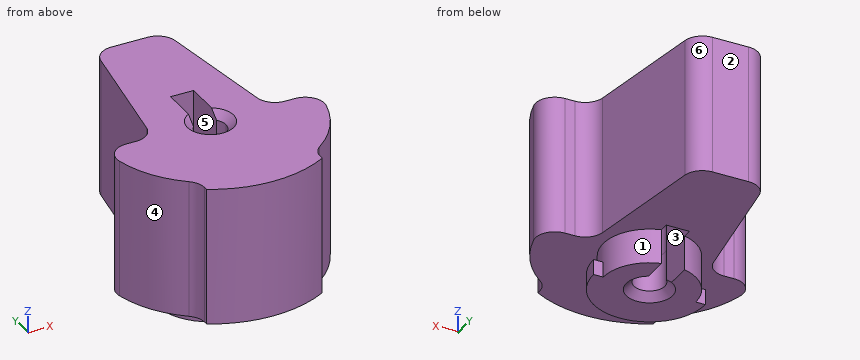
```python
from build123d import *

# Parameters (mm, degrees)
BOSS_EXTRUDE2_DEPTH  = 9.144
CUT_EXTRUDE1_DEPTH   = 0.508
SKETCH4_W            = 1.524
SKETCH4_H            = 3.556
CUT_EXTRUDE2_DEPTH   = 10.144
BOSS_EXTRUDE8_DEPTH  = 9.144
BOSS_EXTRUDE10_DEPTH = 9.144
FILLET2_R            = 1.27
CUT_EXTRUDE4_DEPTH   = 9.144
FILLET4_R            = 1.27
BOSS_EXTRUDE11_DEPTH = 1.27
BOSS_EXTRUDE12_DEPTH = 1.016
BOSS_EXTRUDE13_START = -0.508
BOSS_EXTRUDE13_DEPTH = 0.508
BOSS_EXTRUDE14_DEPTH = 1.27
BOSS_EXTRUDE15_DEPTH = 1.016


with BuildPart() as part:
    # Sketch2 → Boss-Extrude2 (new body)
    with BuildSketch(Plane.XY):
        with BuildLine():
            ThreePointArc((-3.81, 0), (0, -3.81), (3.81, 0))
            Line((3.81, 0), (3.81, 8.636))
            ThreePointArc((3.81, 8.636), (3.363630735, 9.713630735), (2.286, 10.16))
            Line((2.286, 10.16), (-2.286, 10.16))
            ThreePointArc((-2.286, 10.16), (-3.363630735, 9.713630735), (-3.81, 8.636))
            Line((-3.81, 8.636), (-3.81, 0))
        make_face()
        with BuildLine():
            Line((-0.762, 0), (1.016, 0))
            ThreePointArc((1.016, 0), (-0.359210245, -0.950380976), (-0.762, 0.672020833))
            Line((-0.762, 0.672020833), (-0.762, 0))
        make_face(mode=Mode.SUBTRACT)
    extrude(amount=BOSS_EXTRUDE2_DEPTH)

    # Sketch3 → Cut-Extrude1 (cut)
    with BuildSketch(Plane.XY.offset(9.144)):
        with BuildLine():
            Line((-0.762, 0), (1.016, 0))
            ThreePointArc((1.016, 0), (0.950380976, 0.359210245), (0.762, 0.672020833))
            Line((0.762, 0.672020833), (0.762, 3.556))
            Line((0.762, 3.556), (-0.762, 3.556))
            Line((-0.762, 3.556), (-0.762, 0))
        make_face()
    extrude(amount=-CUT_EXTRUDE1_DEPTH, mode=Mode.SUBTRACT)

    # Sketch4 → Cut-Extrude2 (cut, through all)
    with BuildSketch(Plane(origin=(0, 0, 0), x_dir=(-1, 0, 0), z_dir=(0, 0, -1))):
        with Locations((0, 1.778)):
            Rectangle(SKETCH4_W, SKETCH4_H)
    extrude(amount=-CUT_EXTRUDE2_DEPTH, mode=Mode.SUBTRACT)

    # Sketch7 → Cut-Revolve1 (revolve, cut)
    with BuildSketch(Plane(origin=(0, 0, 0), x_dir=(1, 0, 0), z_dir=(0, 1, 0))):
        Polygon((0, 0), (0, -9.144), (1.524, -9.144), (1.016, -8.636), (1.016, -0.508), (1.524, 0), align=None)
    revolve(axis=Axis((0, 0, 0), (0, 0, 1)), mode=Mode.SUBTRACT)

    # Sketch10 → Boss-Extrude8 (add)
    with BuildSketch(Plane.XY.offset(9.144)):
        with BuildLine():
            Line((-3.81, 0), (-6.985, 0))
            ThreePointArc((-6.985, 0), (0, -6.985), (6.985, 0))
            Line((6.985, 0), (3.81, 0))
            ThreePointArc((3.81, 0), (0, -3.81), (-3.81, 0))
        make_face()
    extrude(amount=-BOSS_EXTRUDE8_DEPTH)

    # Sketch14 → Boss-Extrude10 (add)
    with BuildSketch(Plane.XY.offset(9.144)):
        with BuildLine():
            ThreePointArc((3.81, -5.85441073), (0, -6.985), (-3.81, -5.85441073))
            Line((-3.81, -5.85441073), (-3.81, -6.745362036))
            ThreePointArc((-3.81, -6.745362036), (0, -7.747), (3.81, -6.745362036))
            Line((3.81, -6.745362036), (3.81, -5.85441073))
        make_face()
    extrude(amount=-BOSS_EXTRUDE10_DEPTH)

    # Fillet2
    fillet2_edges = [part.edges().sort_by_distance(p)[0] for p in [
        (6.985, 0, 4.572),
        (-6.985, 0, 4.572),
    ]]
    fillet(fillet2_edges, radius=FILLET2_R)

    # Sketch16 → Cut-Extrude4 (cut)
    with BuildSketch(Plane.XY.offset(9.144)):
        with BuildLine():
            Line((-3.81, 0), (-2.286, 10.16))
            ThreePointArc((-2.286, 10.16), (-3.363630735, 9.713630735), (-3.81, 8.636))
            Line((-3.81, 8.636), (-3.81, 0))
        make_face()
        with BuildLine():
            Line((2.286, 10.16), (3.81, 0))
            Line((3.81, 0), (3.81, 8.636))
            ThreePointArc((3.81, 8.636), (3.363630735, 9.713630735), (2.286, 10.16))
        make_face()
    extrude(amount=-CUT_EXTRUDE4_DEPTH, mode=Mode.SUBTRACT)

    # Fillet4
    fillet4_edges = [part.edges().sort_by_distance(p)[0] for p in [
        (-3.81, -5.85441073, 4.572),
        (3.81, -5.85441073, 4.572),
        (-3.81, 0, 4.572),
        (-2.286, 10.16, 4.572),
        (2.286, 10.16, 4.572),
        (3.81, 0, 4.572),
    ]]
    fillet(fillet4_edges, radius=FILLET4_R)

    # Sketch17 → Boss-Extrude11 (add)
    with BuildSketch(Plane(origin=(0, 0, 0), x_dir=(-1, 0, 0), z_dir=(0, 0, -1))):
        with BuildLine():
            Line((0.762, 2.95121331), (0.762, 1.319822715))
            ThreePointArc((0.762, 1.319822715), (0, -1.524), (-0.762, 1.319822715))
            Line((-0.762, 1.319822715), (-0.762, 2.95121331))
            ThreePointArc((-0.762, 2.95121331), (-1.866511184, -2.409655577), (3.048, 0))
            ThreePointArc((3.048, 0), (2.409655577, 1.866511184), (0.762, 2.95121331))
        make_face()
    extrude(amount=BOSS_EXTRUDE11_DEPTH)

    # Sketch18 → Boss-Extrude12 (add)
    with BuildSketch(Plane(origin=(0, 0, -1.27), x_dir=(-1, 0, 0), z_dir=(0, 0, -1))):
        with BuildLine():
            Line((-1.524, 0), (-3.048, 0))
            ThreePointArc((-3.048, 0), (0, -3.048), (3.048, 0))
            Line((3.048, 0), (1.524, 0))
            ThreePointArc((1.524, 0), (0, -1.524), (-1.524, 0))
        make_face()
        with BuildLine():
            Line((-3.048, 0), (-3.683, 0))
            ThreePointArc((-3.683, 0), (0, -3.683), (3.683, 0))
            Line((3.683, 0), (3.048, 0))
            ThreePointArc((3.048, 0), (0, -3.048), (-3.048, 0))
        make_face()
    extrude(amount=BOSS_EXTRUDE12_DEPTH)

    # Sketch20 → Boss-Extrude13 (add)
    with BuildSketch(Plane(origin=(0, 0, 0), x_dir=(-1, 0, 0), z_dir=(0, 0, -1)).offset(BOSS_EXTRUDE13_START)):
        with BuildLine():
            Line((0.762, 1.319822715), (0.762, 0.672020833))
            ThreePointArc((0.762, 0.672020833), (0, -1.016), (-0.762, 0.672020833))
            Line((-0.762, 0.672020833), (-0.762, 1.319822715))
            ThreePointArc((-0.762, 1.319822715), (0, -1.524), (0.762, 1.319822715))
        make_face()
    extrude(amount=BOSS_EXTRUDE13_DEPTH)

    # Sketch21 → Boss-Extrude14 (add)
    with BuildSketch(Plane(origin=(0, 0, 0), x_dir=(-1, 0, 0), z_dir=(0, 0, -1))):
        with BuildLine():
            Line((0.762, 1.319822715), (0.762, 0.672020833))
            ThreePointArc((0.762, 0.672020833), (0, -1.016), (-0.762, 0.672020833))
            Line((-0.762, 0.672020833), (-0.762, 1.319822715))
            ThreePointArc((-0.762, 1.319822715), (0, -1.524), (0.762, 1.319822715))
        make_face()
    extrude(amount=BOSS_EXTRUDE14_DEPTH)

    # Sketch22 → Boss-Extrude15 (add)
    with BuildSketch(Plane(origin=(0, 0, -1.27), x_dir=(-1, 0, 0), z_dir=(0, 0, -1))):
        with BuildLine():
            Line((0.762, 2.95121331), (0.762, 0.672020833))
            ThreePointArc((0.762, 0.672020833), (0, -1.016), (-0.762, 0.672020833))
            Line((-0.762, 0.672020833), (-0.762, 2.95121331))
            ThreePointArc((-0.762, 2.95121331), (-2.409655577, 1.866511184), (-3.048, 0))
            Line((-3.048, 0), (-1.524, 0))
            ThreePointArc((-1.524, 0), (0, -1.524), (1.524, 0))
            Line((1.524, 0), (3.048, 0))
            ThreePointArc((3.048, 0), (2.409655577, 1.866511184), (0.762, 2.95121331))
        make_face()
    extrude(amount=BOSS_EXTRUDE15_DEPTH)

    # Sketch23 → Cut-Revolve2 (revolve, cut)
    with BuildSketch(Plane(origin=(0, 0, 0), x_dir=(1, 0, 0), z_dir=(0, 1, 0))):
        Polygon((0, 2.286), (0, 0), (0.762, 0), (0.762, 1.524), (1.524, 2.286), align=None)
    revolve(axis=Axis((0, 0, -2.286), (0, 0, 1)), mode=Mode.SUBTRACT)


solid = part.part
```
For this review, take the finished solid that the model builds, in its own axes (mm). Face numbers are marked on the shaded views. A direction names the side the tool comes from. Coordinates: 2 decimals unless noted, no trailing zeros. Loops run counter-clockwise (first coordinate to the right, second up) from the corner with the lowest first, then second, coordinate; pieces in that order, holes last. Notation, with made-up numbers: (61, 30) - (81, 30) arc R18 ccw to (81, 65) - close; hole circle Ø1 at (77.5, 74). An arc over 180 degrees is marked (long way). Use one line per item in the form item = value. Start each with the question number.
1) For the marked faces 1 and 2, list the 3-axis set-ups (+Z, -Z, +X, -X, +Y, -Y) from which the entire face can be reached by the end or side of a thin tool; tool diameter is ignored.
2) Take a section at C-C (z = 4.75). State the section outline as (x, y) points (3 decimals).
3) For pin 1 (0.5 mm diameter, centred on x = -5, z = 6, fed in from +Y); pin 2 (1 mm diameter, centred on x = -3, z = 1.5, fed in from -Y); pin 3 (0.7 mm diameter, centred on x = 3, z = -2, fed in from +Y), all flat-tipped, find the tip position at first contact; note any pin that passes through.
4) To check wall thickness, follow probe 1 along X at (y, z) = (0, -0.8); probe 2 along Y at (x, z) = (0, -0.35); probe 3 along Z at (x, y) = (1, -3.75). State the ranges of each line that lie inside material, in increasing order. Write a range as from..to.
5) Draft analysis for pull direction X (two halves, no side actions). For the marked faces 3, 4, 5 and 6, state which applies: released by +X, released by -X, zero draft, split by the parting line, or undercut.
6) Take a section at B-B (y = 3.25). State the section outline as (x, z) points.
7) Take a section at D-D (z = -1.5). State the section outline as (x, y) points, plus the area to 3 significant figures.
8) Take a section at A-A (x = 0). State the section outline as (y, z) points, plus the area to 3 significant figures.
From the geometry:
q1.face_1 = none
q1.face_2 = +Z, -Z, +X, -X, +Y
q2.outline = (-6.81, -1.552) arc R6.985 ccw to (-4.298, -5.506) arc R1.27 cw to (-3.81, -6.507) - (-3.81, -6.745) arc R7.747 ccw to (3.81, -6.745) - (3.81, -6.507) arc R1.27 cw to (4.298, -5.506) arc R6.985 ccw to (6.81, -1.552) arc R1.27 ccw to (5.572, 0) - (4.904, 0) arc R1.27 cw to (3.648, 1.082) - (2.448, 9.078) arc R1.27 ccw to (1.192, 10.16) - (-1.192, 10.16) arc R1.27 ccw to (-2.448, 9.078) - (-3.648, 1.082) arc R1.27 cw to (-4.904, 0) - (-5.572, 0) arc R1.27 ccw to start; hole (-0.762, 0.672) arc R1.016 ccw (long way) to (0.762, 0.672) - (0.762, 3.556) - (-0.762, 3.556) - close
q3.pin_1 = 0.01
q3.pin_2 = -7.33
q3.pin_3 = 1.51
q4.probe_1 = -3.05..-1.02, 1.02..3.05
q4.probe_2 = -3.05..-1.02
q4.probe_3 = 0..9.14
q5.face_3 = undercut
q5.face_4 = released by -X
q5.face_5 = undercut
q5.face_6 = released by +X
q6.outline = (-3.32, 0) - (-0.76, 0) - (-0.76, 9.14) - (-3.32, 9.14) - close; (0.76, 0) - (3.32, 0) - (3.32, 9.14) - (0.76, 9.14) - close
q7.outline = (-3.68, 0) arc R3.68 ccw to (3.68, 0) - (3.05, 0) arc R3.05 ccw to (0.76, 2.95) - (0.76, 0.67) arc R1.02 cw (long way) to (-0.76, 0.67) - (-0.76, 2.95) arc R3.05 ccw to (-3.05, 0) - close
q7.area = 29.4 mm2
q8.outline = (-7.75, 0) - (-3.05, 0) - (-3.05, -1.27) - (-3.68, -1.27) - (-3.68, -2.29) - (-1.52, -2.29) - (-1.02, -1.78) - (-1.02, 8.64) - (-1.52, 9.14) - (-7.75, 9.14) - close; (3.56, 0) - (10.16, 0) - (10.16, 9.14) - (3.56, 9.14) - close
q8.area = 127 mm2
